Read the model definition and answer for the solid it produces. Units are mm, in the model's axes. Face numbers are marked on the shaded views. A direction names the side the tool comes from. Round coordinates to 2 decimals unless told otherwise and drop trailing zeros.
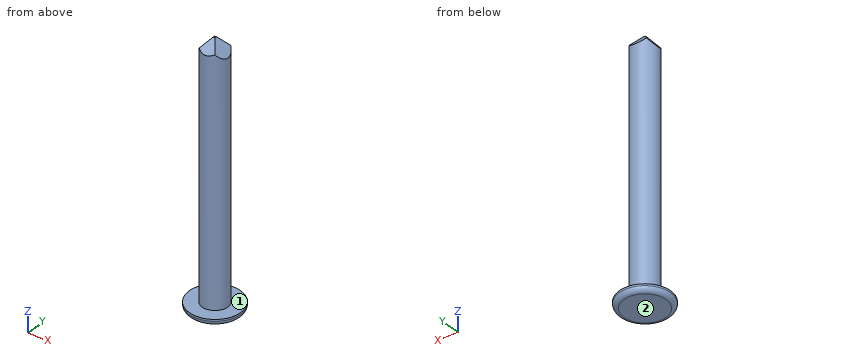
from build123d import *

# Parameters (mm, degrees)
F0_R          = 0.5
F1_DEPTH      = 10
F0_R_2        = 1
F2_DEPTH      = 0.25
F3_R          = 0.18
F5_DEPTH      = 50
F5_DEPTH_BACK = 2.6
F7_DEPTH      = 50
F7_DEPTH_BACK = 2.875


with BuildPart() as f1:
    # F0 (on Top) → F1 (new body)
    with BuildSketch(Plane.XY):
        Circle(F0_R)
    extrude(amount=F1_DEPTH)

    # F0 (on Top) → F2 (join)
    with BuildSketch(Plane.XY):
        Circle(F0_R_2)
        Circle(F0_R, mode=Mode.SUBTRACT)
    extrude(amount=F2_DEPTH)

    # F3
    f3_edges = [f1.edges().sort_by_distance(p)[0] for p in [
        (-1, 0, 0),
    ]]
    fillet(f3_edges, radius=F3_R)

    # F4 (on Front) → F5 (cut, two sides)
    with BuildSketch(Plane.XZ) as f5_sk:
        Polygon((-1.5745003475, 9.1303680092), (-0.7234219229, 9.1651063412), (0, 10.0509226322), (0.7182004047, 9.1477371752), (1.9166575512, 9.1477371752), (1.9166575512, 11.2493792549), (-1.5745003475, 11.2493792549), align=None)
    extrude(amount=-F5_DEPTH, mode=Mode.SUBTRACT)
    extrude(f5_sk.sketch, amount=F5_DEPTH_BACK, mode=Mode.SUBTRACT)

    # F6 (on Right) → F7 (cut, two sides)
    with BuildSketch(Plane.YZ) as f7_sk:
        Polygon((-1.6177080106, 9.4557581469), (-0.6982019986, 9.4029121101), (0, 10.0370543078), (0.6177483219, 9.3569022621), (1.5635710442, 9.3569022621), (1.5635710442, 11.0094053671), (-1.6177080106, 11.0094053671), align=None)
    extrude(amount=-F7_DEPTH, mode=Mode.SUBTRACT)
    extrude(f7_sk.sketch, amount=F7_DEPTH_BACK, mode=Mode.SUBTRACT)


solid = f1.part
Q1. Straight lines are drawn through the part: probe 1 along Z at (x, y) = (-0.25, -0.7); probe 2 along X at (y, z) = (0.05, 1.5); probe 3 along Y at (x, z) = (0.2, 3.25). For each, find the intervals that lie inside material, in ascending order.
Verdict:
probe 1: z = 0 to 0.25
probe 2: x = -0.5 to 0.5
probe 3: y = -0.46 to 0.46
Q2. Which of the six approach directions +Z, -Z, +X, -X, +Y, -Y give full straight-line access (tool end or side, diameter ignored) to the marked faces 1 and 2?
Verdict:
face 1: +Z
face 2: -Z, +X, -X, +Y, -Y
Q3. A flat-ended cylindrical pin translates along its axis: pin 1 Ø1 at (x, y) = (0, -0.5) entering from +Z. Find the tip coordinate at first contact, or state that the pin passes through.
Verdict:
pin 1: stops at z = 10
